```python
from build123d import *

# Parameters (mm, degrees)
SKETCH1_R           = 3.3655
SKETCH1_R_2         = 11.571823904
SKETCH1_R_3         = 4.191
SKETCH1_R_4         = 7.8105
BOSS_EXTRUDE1_DEPTH = 3.175


with BuildPart() as part:
    # Sketch1 → Boss-Extrude1 (new body)
    # profile 1 of 7: a face of its own
    with BuildSketch(Plane.XY):
        with BuildLine():
            ThreePointArc((-13.801669145, -2.162135242), (-13.92785371, -1.084338979), (-13.97, 0))
            Line((-13.97, 0), (-10.16, 137.668))
            ThreePointArc((-10.16, 137.668), (-9.861385845, 140.113131739), (-8.98309661, 142.414532976))
            Line((-8.98309661, 142.414532976), (-49.565953559, 65.609056962))
            ThreePointArc((-49.565953559, 65.609056962), (-50.742856949, 60.862523985), (-49.565953559, 56.115991009))
            Line((-49.565953559, 56.115991009), (-13.801669145, -2.162135242))
        make_face()
        with Locations((-40.582856949, 60.862523985)):
            Circle(SKETCH1_R, mode=Mode.SUBTRACT)
    # profile 2 of 7: a face of its own
    with BuildSketch(Plane.XY):
        with BuildLine():
            Line((49.565953559, 65.609056962), (8.98309661, 142.414532976))
            ThreePointArc((8.98309661, 142.414532976), (9.861385845, 140.113131739), (10.16, 137.668))
            Line((10.16, 137.668), (13.97, 0))
            ThreePointArc((13.97, 0), (13.92785371, -1.084338979), (13.801669145, -2.162135242))
            Line((13.801669145, -2.162135242), (49.565953559, 56.115991009))
            ThreePointArc((49.565953559, 56.115991009), (50.742856949, 60.862523985), (49.565953559, 65.609056962))
        make_face()
        with Locations((40.582856949, 60.862523985)):
            Circle(SKETCH1_R, mode=Mode.SUBTRACT)
    # profile 3 of 7: a face of its own
    with BuildSketch(Plane.XY):
        with BuildLine():
            ThreePointArc((-10.16, 137.668), (7.886144716, 68.281846548), (-13.97, 0))
            ThreePointArc((-13.97, 0), (-13.92785371, -1.084338979), (-13.801669145, -2.162135242))
            Line((-13.801669145, -2.162135242), (-8.177790267, -11.326281223))
            ThreePointArc((-8.177790267, -11.326281223), (0, -13.97), (8.177790267, -11.326281223))
            Line((8.177790267, -11.326281223), (13.801669145, -2.162135242))
            ThreePointArc((13.801669145, -2.162135242), (13.92785371, -1.084338979), (13.97, 0))
            Line((13.97, 0), (10.16, 137.668))
            ThreePointArc((10.16, 137.668), (9.861385845, 140.113131739), (8.98309661, 142.414532976))
            ThreePointArc((8.98309661, 142.414532976), (0, 147.828), (-8.98309661, 142.414532976))
            ThreePointArc((-8.98309661, 142.414532976), (-9.861385845, 140.113131739), (-10.16, 137.668))
        make_face()
        Circle(SKETCH1_R_2, mode=Mode.SUBTRACT)
        with Locations((0, 137.668)):
            Circle(SKETCH1_R_3, mode=Mode.SUBTRACT)
    # profile 4 of 7: a face of its own
    with BuildSketch(Plane.XY):
        with BuildLine():
            ThreePointArc((-10.16, 137.668), (7.886144716, 68.281846548), (-13.97, 0))
            Line((-13.97, 0), (-10.16, 137.668))
        make_face()
    # profile 5 of 7: a face of its own
    with BuildSketch(Plane.XY):
        with BuildLine():
            Line((13.801669145, -2.162135242), (8.177790267, -11.326281223))
            ThreePointArc((8.177790267, -11.326281223), (11.906701974, -7.306938353), (13.801669145, -2.162135242))
        make_face()
    # profile 6 of 7: a face of its own
    with BuildSketch(Plane.XY):
        with BuildLine():
            Line((-8.177790267, -11.326281223), (-13.801669145, -2.162135242))
            ThreePointArc((-13.801669145, -2.162135242), (-11.906701974, -7.306938353), (-8.177790267, -11.326281223))
        make_face()
    # profile 7 of 7: a face of its own
    with BuildSketch(Plane.XY):
        Circle(SKETCH1_R_2)
        Circle(SKETCH1_R_4, mode=Mode.SUBTRACT)
    extrude(amount=BOSS_EXTRUDE1_DEPTH)


solid = part.part
```
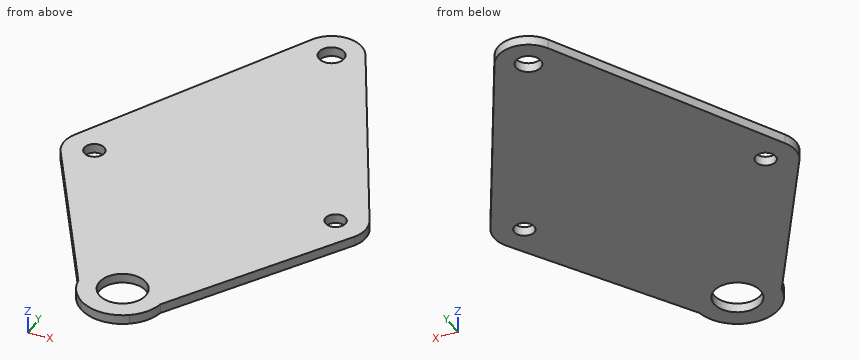
Input: part model. Units: mm. Frame: model coordinates. Give positions to 0.01 mm unless a question says otherwise; leave off trailing zeros. Order: outer loops, then holes, each group sorted by start corner. A loop starts at its lowest first (then second) coordinate and runs counter-clockwise, first axis right, second up. Notation, with made-up numbers: M 77,47 L 83,47 A18 cw 83,55 Z; hole C -19,62.5 d8. An arc over 180 degrees is marked long. One line per question, with ' | ' between items. Start each with the question number.
1. Section query A-A (x = 0). Return the cut outline in (y, z) (1 decimal), and give its area (4 significant figures).
2. Section query C-C (z = 2.3). Return the cut outline in (x, y).
3. Section query B-B (y = 0). Return the cut outline in (x, z) (1 decimal), and give its area (3 significant figures).
4. Section query D-D (y = 69). Return the cut outline in (x, z) (3 decimals).
5. Material intervals for probe 1 along Y at (x, z) = (0, 0.85); probe 2 along Y at (x, z) = (-2, 2.75) (3 decimals); probe 3 along X at (y, z) = (136, 2.45), sorted ascending. Write a range as [from, to].
Here are the results:
1) outline: M -14,0 L -7.8,0 L -7.8,3.2 L -14,3.2 Z; M 7.8,0 L 133.5,0 L 133.5,3.2 L 7.8,3.2 Z; M 141.9,0 L 147.8,0 L 147.8,3.2 L 141.9,3.2 Z | area: 437.5 mm²
2) outline: M -49.57,56.12 L -13.8,-2.16 A13.97 ccw 13.8,-2.16 L 49.57,56.12 A10.16 ccw 49.57,65.61 L 8.98,142.41 A10.16 ccw -8.98,142.41 L -49.57,65.61 A10.16 ccw Z; hole C -40.58,60.86 d6.73; hole C 0,0 d15.62; hole C 0,137.67 d8.38; hole C 40.58,60.86 d6.73
3) outline: M -15.1,0 L -7.8,0 L -7.8,3.2 L -15.1,3.2 Z; M 7.8,0 L 15.1,0 L 15.1,3.2 L 7.8,3.2 Z | area: 46.5 mm²
4) outline: M -47.774,0 L 47.774,0 L 47.774,3.175 L -47.774,3.175 Z
5) probe 1: [-13.97, -7.81], [7.81, 133.48], [141.86, 147.83] | probe 2: [-13.826, -7.55], [7.55, 133.985], [141.351, 147.629] | probe 3: [-12.37, -3.84], [3.84, 12.37]
